Design review of the part built by this model. Coordinates are the model's own, in mm. Face numbers are marked on the shaded views. A direction names the side the tool comes from. Coordinates: 2 decimals unless noted, no trailing zeros. Loops run counter-clockwise (first coordinate to the right, second up) from the corner with the lowest first, then second, coordinate; pieces in that order, holes last.
Q1. Add section A-A on z = 7.62. Give the number of separate pieces and of enclosed holes in the cut face, and give its area (3 significant figures).
Q2. Machinability: for the marked faces 5 and 6, which of the approach directions +Z, -Z, +X, -X, +Y, -Y give a long, thin tool a straight path to every point of the face, cutting with its end or side? Answer none if there is none.
Q3. Draft analysis for pull direction Z (two halves, no side actions). For the marked faces 1, 2, 3 and 4, state which applies: released by +Z, released by -Z, zero draft, split by the parting line, or undercut.
Q4. Add section C-C on x = -10.5. Give the boundary of the cut face in (y, z).
Q5. Wall thickness on probe 1 along X at (y, z) = (-7.5, 7.62); probe 2 along X at (y, z) = (-8, 7); probe 3 along Z at (x, y) = (-5.5, 10): over which ranges is each line inside the solid? List them lowest first.
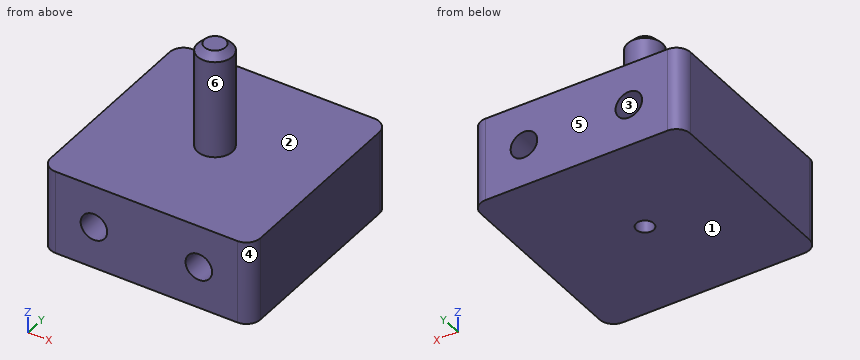
```python
from build123d import *

# Parameters (mm, degrees)
SKETCH1_W           = 38.1
SKETCH1_H           = 38.1
SKETCH1_R           = 1.5875
BOSS_EXTRUDE2_DEPTH = 15.24
SKETCH3_R           = 3.175
BOSS_EXTRUDE3_DEPTH = 19.05
FILLET2_R           = 2.54
CHAMFER1_SIZE       = 1.27
SKETCH4_R           = 2.413
CUT_EXTRUDE2_DEPTH  = 7.62
SKETCH5_R           = 2.413
CUT_EXTRUDE3_DEPTH  = 7.62
SKETCH6_R           = 2.413
CUT_EXTRUDE4_DEPTH  = 39.1


with BuildPart() as part:
    # Sketch1 → Boss-Extrude2 (new body)
    with BuildSketch(Plane.XY):
        Rectangle(SKETCH1_W, SKETCH1_H)
        Circle(SKETCH1_R, mode=Mode.SUBTRACT)
    extrude(amount=BOSS_EXTRUDE2_DEPTH)

    # Sketch3 → Boss-Extrude3 (add)
    with BuildSketch(Plane.XY.offset(15.24)):
        Circle(SKETCH3_R)
    extrude(amount=BOSS_EXTRUDE3_DEPTH)

    # Fillet2
    fillet2_edges = [part.edges().sort_by_distance(p)[0] for p in [
        (-19.05, 19.05, 7.62),
        (19.05, 19.05, 7.62),
        (19.05, -19.05, 7.62),
        (-19.05, -19.05, 7.62),
    ]]
    fillet(fillet2_edges, radius=FILLET2_R)

    # Chamfer1
    chamfer1_edges = [part.edges().sort_by_distance(p)[0] for p in [
        (-3.175, 0, 34.29),
    ]]
    chamfer(chamfer1_edges, length=CHAMFER1_SIZE)

    # Sketch4 → Cut-Extrude2 (cut)
    with BuildSketch(Plane.XZ.offset(19.05)):
        with Locations((-9.525, 7.62)):
            Circle(SKETCH4_R)
        with Locations((9.525, 7.62)):
            Circle(SKETCH4_R)
    extrude(amount=-CUT_EXTRUDE2_DEPTH, mode=Mode.SUBTRACT)

    # Sketch5 → Cut-Extrude3 (cut)
    with BuildSketch(Plane(origin=(0, 19.05, 0), x_dir=(1, 0, 0), z_dir=(0, 1, 0))):
        with Locations((9.525, -7.62)):
            Circle(SKETCH5_R)
        with Locations((-9.525, -7.62)):
            Circle(SKETCH5_R)
    extrude(amount=-CUT_EXTRUDE3_DEPTH, mode=Mode.SUBTRACT)

    # Sketch6 → Cut-Extrude4 (cut, through all)
    with BuildSketch(Plane(origin=(0, 19.05, 0), x_dir=(1, 0, 0), z_dir=(0, 1, 0))):
        with Locations((9.525, -7.62)):
            Circle(SKETCH6_R)
        with Locations((-9.525, -7.62)):
            Circle(SKETCH6_R)
    extrude(amount=-CUT_EXTRUDE4_DEPTH, mode=Mode.SUBTRACT)


solid = part.part
```
Entries:
1. separate pieces: 3
1. enclosed holes: 1
1. area: 1,070 mm2
2. face 5: +Z, -Z, +X, -X, +Y
2. face 6: +Z
3. face 1: released by -Z
3. face 2: released by +Z
3. face 3: undercut
3. face 4: zero draft
4. outline: (-19.05, 0) - (19.05, 0) - (19.05, 5.41) - (-19.05, 5.41) - close; (-19.05, 9.83) - (19.05, 9.83) - (19.05, 15.24) - (-19.05, 15.24) - close
5. probe 1: x = -19.05 to -11.94, -7.11 to 7.11, 11.94 to 19.05
5. probe 2: x = -19.05 to -11.86, -7.19 to 7.19, 11.86 to 19.05
5. probe 3: z = 0 to 15.24
